```python
from build123d import *

# Parameters (mm, degrees)
F0_R      = 31.75
F1_DEPTH  = 50.8
F1_FACE_R = 31.75
F2_DEPTH  = 50.8
F3_R      = 27.939053
F4_DEPTH  = 50.8
F4_FACE_R = 27.939053
F5_DEPTH  = 50.8


with BuildPart() as f1:
    # F0 (on Front) → F1 (new body)
    with BuildSketch(Plane.XZ):
        Circle(F0_R)
    extrude(amount=-F1_DEPTH)

    # F1_face (on face) → F2 (join)
    with BuildSketch(Plane.XZ):
        Circle(F1_FACE_R)
    extrude(amount=F2_DEPTH)

    # F3 (on Front) → F4 (cut)
    with BuildSketch(Plane.XZ):
        Circle(F3_R)
    extrude(amount=-F4_DEPTH, mode=Mode.SUBTRACT)

    # F4_face (on face) → F5 (cut)
    with BuildSketch(Plane(origin=(0, 0, 0), x_dir=(1, 0, 0), z_dir=(0, 1, 0))):
        Circle(F4_FACE_R)
    extrude(amount=-F5_DEPTH, mode=Mode.SUBTRACT)


solid = f1.part
```
Source: CAD feature listing. Evaluate the final solid. Frame: model axes, mm. Coordinates: 2 decimals unless noted, no trailing zeros. Order: outer loops, then holes, each group sorted by start corner. A loop starts at its lowest first (then second) coordinate and runs counter-clockwise, first axis right, second up. Notation, with made-up numbers: (32.25, 63.25) - (55.25, 63.25) arc R15 cw to (55.25, 86.25) - close; hole circle Ø5 at (-2, 59.25). An arc over 180 degrees is marked (long way). One line per item, written item: value.
1) Cut plane B-B on x = 0. Output: boundary loops of the cut face in (y, z).
Computed values:
outline: (-50.8, -31.75) - (50.8, -31.75) - (50.8, -27.94) - (-50.8, -27.94) - close; (-50.8, 27.94) - (50.8, 27.94) - (50.8, 31.75) - (-50.8, 31.75) - close
2) Contact query for flat-ended pins moving along their axis: pin 1 (1.5 mm diameter, centred on y = -9.5, z = -9, fed in from -X); pin 2 (1.5 mm diameter, centred on y = -12, z = 25, fed in from +X); pin 3 (10 mm diameter, centred on x = -8, y = 13, fed in from -Z). Output: stop coordinate, or through.
Computed values:
pin 1: stops at x = -30.66
pin 2: stops at x = 20.49
pin 3: stops at z = -31.61
3) Ray query, line 1 (X direction, y = 8, z = 1); line 2 (Z direction, x = 0, y = -13); line 3 (Z direction, x = -15, y = 30). Return the intervals inside material, ascending. Write a range as [from, to].
Computed values:
line 1: x = [-31.73, -27.92], [27.92, 31.73]
line 2: z = [-31.75, -27.94], [27.94, 31.75]
line 3: z = [-27.98, -23.57], [23.57, 27.98]
4) Cut plane A-A on z = 0. Output: boundary loops of the cut face in (x, y), plus the area to 3 significant figures.
Computed values:
outline: (-31.75, -50.8) - (-27.94, -50.8) - (-27.94, 50.8) - (-31.75, 50.8) - close; (27.94, -50.8) - (31.75, -50.8) - (31.75, 50.8) - (27.94, 50.8) - close
area: 774 mm^2
5) Cut plane C-C on y = -44. Output: boundary loops of the cut face in (x, z), plus the area to 3 significant figures.
Computed values:
outline: circle Ø63.5 at (0, 0); hole circle Ø55.88 at (0, 0)
area: 715 mm^2
